CAD build for the part. Positions are in the model's coordinates, mm. A direction names the side the tool comes from. Coordinates: 2 decimals unless noted, no trailing zeros. Order: outer loops, then holes, each group sorted by start corner. A loop starts at its lowest first (then second) coordinate and runs counter-clockwise, first axis right, second up. Notation, with made-up numbers: (58.5, 52.5) - (72.5, 52.5) arc R21 cw to (72.5, 75.5) - close; hole circle Ø2 at (62.25, 31.5). An arc over 180 degrees is marked (long way). Return JSON: item names as keys, results as strings.
from build123d import *

# Parameters (mm, degrees)
SKETCH_1_R      = 2.5
EXTRUDE_1_DEPTH = 2
SKETCH_2_R      = 2
EXTRUDE_3_DEPTH = 2
EXTRUDE_4_REACH = 90.577
SKETCH_4_R      = 2.5


with BuildPart() as part:
    # Sketch 1 → Extrude 1 (new body)
    with BuildSketch(Plane(origin=(0, 0, 0), x_dir=(1, 0, 0), z_dir=(0, 1, 0))):
        Polygon((17.573593129, -60), (60, -17.573593129), (60, 0), (20, 0), (20, -20), (0, -20), (0, -60), align=None)
        with Locations(Location((10, -52, 0), (0, 0, 270))):
            Circle(SKETCH_1_R, mode=Mode.SUBTRACT)
        with Locations(Location((52, -10, 0), (0, 0, 270))):
            Circle(SKETCH_1_R, mode=Mode.SUBTRACT)
    extrude(amount=EXTRUDE_1_DEPTH)



with BuildPart() as body_2:
    # Sketch 2 → Extrude 3 (new body)
    with BuildSketch(Plane(origin=(20.100505063, 28.426406871, 20.100505063), x_dir=(-0.7071067811865476, 0, 0.7071067811865476), z_dir=(0.5000000000000009, 0.7071067811865465, 0.5000000000000009))):
        Polygon((-3, 33.431239936), (-15, 33.431239936), (-15, 3.431239936), (15, 3.431239936), (15, 28.431239936), (11, 28.431239936), (-3, 28.431239936), align=None)
        with Locations(Location((-11, 6.431239936, 0), (0, 0, 54.735610317))):
            Circle(SKETCH_2_R, mode=Mode.SUBTRACT)
        with Locations(Location((11, 6.431239936, 0), (0, 0, 54.735610317))):
            Circle(SKETCH_2_R, mode=Mode.SUBTRACT)
        with Locations(Location((-11, 30.431239936, 0), (0, 0, 54.735610317))):
            Circle(SKETCH_2_R, mode=Mode.SUBTRACT)
    extrude(amount=EXTRUDE_3_DEPTH)


with BuildPart() as part_1:
    add(part.part)

    add(body_2.part)  # Extrude 4 merges body 2
    # Extrude 4: up to this plane
    extrude_4_end = Plane(origin=(20.100505063, 28.426406871, 20.100505063), z_dir=(0.5000000000000009, 0.7071067811865464, 0.5000000000000009))
    # Sketch 4 → Extrude 4 (add, up to the surface)
    with BuildSketch(Plane(origin=(0, 2, 0), x_dir=(1, 0, 0), z_dir=(0, 1, 0)), mode=Mode.PRIVATE) as extrude_4_sk1:
        with Locations(Location((30.42692979, -27.445922357, 0), (0, 0, 315))):
            Circle(SKETCH_4_R)
    extrude_4_tool1 = split(extrude(extrude_4_sk1.sketch, amount=EXTRUDE_4_REACH, mode=Mode.PRIVATE), bisect_by=extrude_4_end, keep=Keep.BOTH, mode=Mode.PRIVATE)
    add(extrude_4_tool1.solids().sort_by_distance((30.42693, 2, 27.445922))[0])


solid = part_1.part
Item 1: Which spindle directions (+Z, -Z, +X, -X, +Y, -Y) get a long thin tool onto all of the face, cutting with end or side? Do faces 4 (the flat face through (43.61, 5.48, 31)), 5 (the flat face through (20, 1, 10)), 6 (the flat face through (38.16, 7.28, 33.92)), 7 (the flat face through (17.865, 17.982, 39.078)), 8 (the cylindrical face through (28.74, 8.31, 25.6)). Say none if no direction does.
Findings below:
{"face 4": "+Z, +X", "face 5": "-Z, -X, +Y, -Y", "face 6": "+Z", "face 7": "+Z, -X, +Y", "face 8": "none"}
Item 2: Band-saw the part on C-C, the plane y = 15.75. List the corners of the cut face in (x, z).
Findings below:
{"outline": "(18.46, 39.67) - (28.79, 29.34) arc R2.5 ccw (long way) to (32.32, 25.81) - (39.67, 18.46) - (41.67, 20.46) - (20.46, 41.67) - close"}
Item 3: Band-saw the part on A-A, the plane z = 10. List the corners of the cut face in (x, y), then the cut area to 3 significant figures.
Findings below:
{"outline": "(20, 0) - (49.5, 0) - (49.5, 2) - (20, 2) - close; (54.5, 0) - (60, 0) - (60, 2) - (54.5, 2) - close", "area": "70.0 mm²"}
Item 4: Mould opens along Y. For faces 1 (the flat face through (40.521, 15.942, 19.308)), 2 (the flat face through (23, 2, 30)), 3 (the flat face through (30, 0, 30)) say: released by +Y, released by -Y, zero draft, split by the parting line, or undercut.
Findings below:
{"face 1": "zero draft", "face 2": "undercut", "face 3": "released by -Y"}
Item 5: Drop flat-ended pins along their axis: P1, Ø4, axis at x = 52, z = 10, coming from the +Y side; P2, Ø2, axis at x = 11.5, y = 1, coming from the -Z side; P3, Ø1.6, axis at y = 1, z = 7.5, coming from the -X side; P4, Ø2, axis at x = 33.5, z = 15, coming from the +Y side. Give the stop position or say it passes through.
Findings below:
{"P1": "passes through", "P2": "stops at z = 20", "P3": "stops at x = 20", "P4": "stops at y = 26.39"}
Item 6: Band-saw the part on D-D, the plane y = 19.5. List the corners of the cut face in (x, z), then the cut area to 3 significant figures.
Findings below:
{"outline": "(15.81, 37.02) - (37.02, 15.81) - (39.02, 17.81) - (17.81, 39.02) - close", "area": "84.9 mm²"}
Item 7: Wall check: L1, parallel to Y at x = 8.5, z = 24; L2, parallel to X at y = 0.8, z = 52; L3, parallel to X at y = 11, z = 43. Give the ranges that are in metal, low to high. Write a range as [from, to].
Findings below:
{"L1": "y = [0, 2]", "L2": "x = [0, 7.5], [12.5, 25.57]", "L3": "x = [21.85, 25.85]"}
Item 8: Band-saw the part on B-B, the plane x = 10. List the corners of the cut face in (y, z).
Findings below:
{"outline": "(0, 20) - (2, 20) - (2, 49.5) - (0, 49.5) - close; (0, 54.5) - (2, 54.5) - (2, 60) - (0, 60) - close"}
